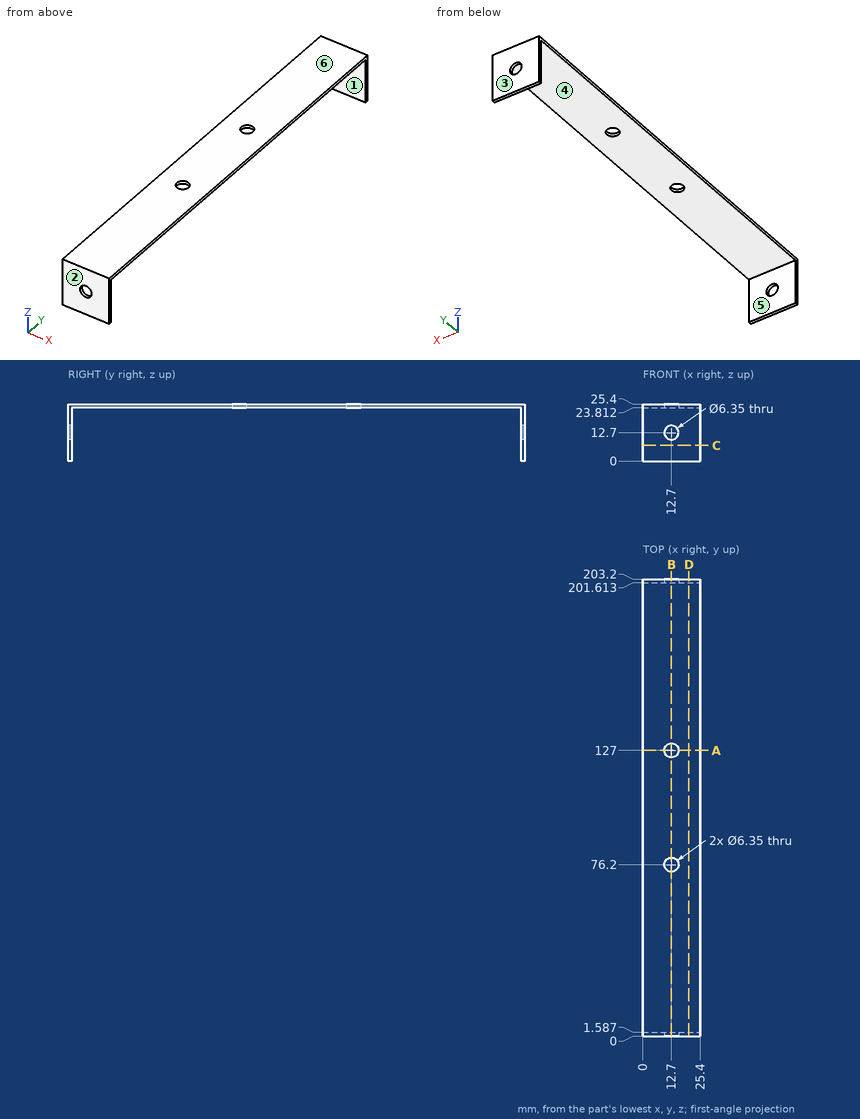
Input: dimensioned drawing with shaded views. Units: mm. Origin: part minimum x, y, z. A direction names the side the tool comes from. Give positions to 0.01 mm unless a question says otherwise; leave off trailing zeros. Loops run counter-clockwise (first coordinate to the right, second up) from the corner with the lowest first, then second, coordinate; pieces in that order, holes last. Notation, with made-up numbers: (-2.75, -16) - (9.25, -16) arc R23 ccw to (9.25, 14) - close; hole circle Ø9 at (-12.5, 57). An arc over 180 degrees is marked (long way). Answer as CSV lines item,"result". Start each with the question number.
(1) Section query B-B (x = 12.7). Output: boundary loops of the cut face in (y, z) (1 decimal).
(2) Section query D-D (x = 20.5). Output: boundary loops of the cut face in (y, z).
(3) Ray query, line 1 along Y through (x, z) = (12.7, 24.7) (1 decimal); line 2 along Z through (x, y) = (12.7, 202.6) (1 decimal); line 3 along Y through (x, z) = (11.25, 16). Return the intervals inside material, ascending. Write a range as [from, to].
(4) Section query A-A (y = 127). Output: boundary loops of the cut face in (x, z) (1 decimal).
(5) Reachability of the marked faces 1 and 2 from +Z, -Z, +X, -X, +Y, -Y: full face, straight path, thin tool, end or side. Return the list, or none.
(6) Section query C-C (z = 7). Output: boundary loops of the cut face in (x, y).
(7) Pin query (flat end, axial travel): P1, Ø5.5, axis at x = 12.7, z = 12.7, coming from the +Y side; P2, Ø8.5, axis at x = 12.7, y = 127, coming from the -Z side. Return the tip coordinate at first contact, or that it passes through.
(8) Mould query, pull axis Y, two halves, no side actions, for the marked faces 3, 4, 5 and 6. Classes: +Y half, -Y half, draft (parallel to the pull), parting line (faces both ways), or undercut.
Worked answers:
1,outline,"(0, 0) - (1.6, 0) - (1.6, 9.5) - (0, 9.5) - close; (0, 15.9) - (1.6, 15.9) - (1.6, 23.8) - (73, 23.8) - (73, 25.4) - (0, 25.4) - close; (79.4, 23.8) - (123.8, 23.8) - (123.8, 25.4) - (79.4, 25.4) - close; (130.2, 23.8) - (201.6, 23.8) - (201.6, 15.9) - (203.2, 15.9) - (203.2, 25.4) - (130.2, 25.4) - close; (201.6, 0) - (203.2, 0) - (203.2, 9.5) - (201.6, 9.5) - close"
2,outline,"(0, 0) - (1.59, 0) - (1.59, 23.81) - (201.61, 23.81) - (201.61, 0) - (203.2, 0) - (203.2, 25.4) - (0, 25.4) - close"
3,line 1,"y = [0, 73], [79.4, 123.8], [130.2, 203.2]"
3,line 2,"z = [0, 9.5], [15.9, 25.4]"
3,line 3,"y = [0, 1.59], [201.61, 203.2]"
4,outline,"(0, 23.8) - (9.5, 23.8) - (9.5, 25.4) - (0, 25.4) - close; (15.9, 23.8) - (25.4, 23.8) - (25.4, 25.4) - (15.9, 25.4) - close"
5,face 1,"-Z, +X, -X"
5,face 2,"+Z, -Z, +X, -X, -Y"
6,outline,"(0, 0) - (25.4, 0) - (25.4, 1.59) - (0, 1.59) - close; (0, 201.61) - (25.4, 201.61) - (25.4, 203.2) - (0, 203.2) - close"
7,P1,"passes through"
7,P2,"stops at z = 23.81"
8,face 3,"+Y half"
8,face 4,"undercut"
8,face 5,"undercut"
8,face 6,"draft"
